```python
from build123d import *

# Parameters (mm, degrees)
F0_W          = 73
F0_H          = 73
F0_W_2        = 56
F0_H_2        = 56
F0_W_3        = 52
F0_H_3        = 52
F1_DEPTH      = 20
F0_W_4        = 76
F0_H_4        = 76
F2_DEPTH      = 3
F3_DEPTH      = 10
F4_W          = 10
F4_H          = 5
F5_DEPTH      = 80
F6_W          = 5
F6_H          = 10
F7_DEPTH      = 80
F8_W          = 8
F8_H          = 5
F9_DEPTH      = 80
F10_W         = 5
F10_H         = 8
F11_DEPTH     = 80
F12_SIZE      = 1
F13_T         = 2.5
F13_T3_DEPTH  = 62
F13_T5_DEPTH  = 62
F13_T7_DEPTH  = 78
F13_T9_DEPTH  = 78
F13_T11_DEPTH = 25


# Not quite as in the source:
# - a shell that OpenCascade refuses in one call is made with other operations: the cavity is built on its own and cut out


with BuildPart() as f1:
    # F0 (on Front) → F1 (new body)
    with BuildSketch(Plane.XZ):
        with Locations((38, 38)):
            Rectangle(F0_W, F0_H)
        with Locations((38, 38)):
            Rectangle(F0_W_2, F0_H_2, mode=Mode.SUBTRACT)
        with Locations((38, 38)):
            Rectangle(F0_W_2, F0_H_2)
        with Locations((38, 38)):
            Rectangle(F0_W_3, F0_H_3, mode=Mode.SUBTRACT)
    extrude(amount=F1_DEPTH)

    # F0 (on Front) → F2 (join)
    with BuildSketch(Plane.XZ):
        with Locations((38, 38)):
            Rectangle(F0_W_4, F0_H_4)
        with Locations((38, 38)):
            Rectangle(F0_W, F0_H, mode=Mode.SUBTRACT)
    extrude(amount=F2_DEPTH)

    # F0 (on Front) → F3 (join)
    with BuildSketch(Plane.XZ):
        with Locations((38, 38)):
            Rectangle(F0_W_4, F0_H_4)
        with Locations((38, 38)):
            Rectangle(F0_W, F0_H, mode=Mode.SUBTRACT)
    extrude(amount=F3_DEPTH)

    # F4 (on Top) → F5 (cut)
    with BuildSketch(Plane.XY):
        with Locations((5, -2.5)):
            Rectangle(F4_W, F4_H)
        with Locations((71, -2.5)):
            Rectangle(F4_W, F4_H)
    extrude(amount=F5_DEPTH, mode=Mode.SUBTRACT)

    # F6 (on Right) → F7 (cut)
    with BuildSketch(Plane.YZ):
        with Locations((-2.5, 5)):
            Rectangle(F6_W, F6_H)
        with Locations((-2.5, 71)):
            Rectangle(F6_W, F6_H)
    extrude(amount=F7_DEPTH, mode=Mode.SUBTRACT)

    # F8 (on Top) → F9 (cut)
    with BuildSketch(Plane.XY):
        with Locations((5.5, -17.5)):
            Rectangle(F8_W, F8_H)
        with Locations((70.5, -17.5)):
            Rectangle(F8_W, F8_H)
    extrude(amount=F9_DEPTH, mode=Mode.SUBTRACT)

    # F10 (on Right) → F11 (cut)
    with BuildSketch(Plane.YZ):
        with Locations((-17.5, 5.5)):
            Rectangle(F10_W, F10_H)
        with Locations((-17.5, 70.5)):
            Rectangle(F10_W, F10_H)
    extrude(amount=F11_DEPTH, mode=Mode.SUBTRACT)

    # F12
    f12_edges = [f1.edges().sort_by_distance(p)[0] for p in [
        (38, -10, 0),
        (0, -10, 38),
        (76, -10, 38),
        (38, -10, 76),
        (66.5, -20, 38),
        (38, -20, 66.5),
        (38, -20, 9.5),
        (9.5, -20, 38),
    ]]
    chamfer(f12_edges, length=F12_SIZE)

    # F13: shell of thickness 2.5, made by hand


with BuildPart() as f13_core1:
    # F13_t2: copy of F1
    add(f1.part)

    # the walls: a layer under each face that stays
    f13_faces = [f13_core1.faces().sort_by_distance(p)[0] for p in [
        (9.5, -17, 38),
        (38, -17, 66.5),
        (10, -19.5, 38),
        (69.2857142857, -15, 69.2857142857),
        (38, -17, 9.5),
        (38, -19.5, 66),
        (66.5, -17, 38),
        (38, -19.5, 10),
        (56.90625, -20, 11.1790123457),
        (1.5, -12.5, 38),
        (38, -12.5, 1.5),
        (74.5, -12.5, 38),
        (38, -12.5, 74.5),
        (66, -19.5, 38),
        (64, -10, 38),
        (38, -10, 64),
        (38, -10, 12),
        (12, -10, 38),
        (40.890625, -10, 1.304526749),
        (11.8666666667, 0, 11.8666666667),
        (38, -9.5, 0.5),
        (0.5, -9.5, 38),
        (75.5, -9.5, 38),
        (38, -9.5, 75.5),
        (66, -2.5, 38),
        (38, -2.5, 10),
        (10, -2.5, 38),
        (38, -2.5, 66),
        (38, -7, 0),
        (0, -7, 38),
        (76, -7, 38),
        (38, -7, 76),
    ]]
    thicken(f13_faces, amount=-F13_T, mode=Mode.SUBTRACT)

    # F13_s4 → F13_t3 (cut)
    with BuildSketch(Plane.XY.offset(7)):
        Polygon((9.475, -15.025), (12, -15), (12, -12.5), (9.5, -12.5), align=None)
        Polygon((66.525, -15.025), (66.5, -12.5), (64, -12.5), (64, -15), align=None)
    extrude(amount=F13_T3_DEPTH, mode=Mode.SUBTRACT)

    # F13_s6 → F13_t5 (cut)
    with BuildSketch(Plane.YZ.offset(7)):
        Polygon((-15.025, 66.525), (-15, 64), (-12.5, 64), (-12.5, 66.5), align=None)
        Polygon((-15.025, 9.475), (-12.5, 9.5), (-12.5, 12), (-15, 12), align=None)
    extrude(amount=F13_T5_DEPTH, mode=Mode.SUBTRACT)

    # F13_s8 → F13_t7 (cut)
    with BuildSketch(Plane.XY.offset(-1)):
        Polygon((1.475, -10.025), (4, -10), (4, -7.5), (1.5, -7.5), align=None)
        Polygon((74.525, -10.025), (72, -10), (72, -7.5), (74.5, -7.5), align=None)
    extrude(amount=F13_T7_DEPTH, mode=Mode.SUBTRACT)

    # F13_s10 → F13_t9 (cut)
    with BuildSketch(Plane.YZ.offset(-1)):
        Polygon((-10.025, 1.475), (-10, 4), (-7.5, 4), (-7.5, 1.5), align=None)
        Polygon((-10.025, 74.525), (-10, 72), (-7.5, 72), (-7.5, 74.5), align=None)
    extrude(amount=F13_T9_DEPTH, mode=Mode.SUBTRACT)

    # F13_s12 → F13_t11 (cut)
    with BuildSketch(Plane.XZ.offset(-2.5)):
        Polygon((63.975, 63.975), (66.5, 64), (66.5, 66.5), (64, 66.5), align=None)
        Polygon((63.975, 12.025), (66.5, 12), (66.5, 9.5), (64, 9.5), align=None)
        Polygon((12.025, 63.975), (12, 66.5), (9.5, 66.5), (9.5, 64), align=None)
        Polygon((12.025, 12.025), (12, 9.5), (9.5, 9.5), (9.5, 12), align=None)
    extrude(amount=F13_T11_DEPTH, mode=Mode.SUBTRACT)


with BuildPart() as f1_1:
    add(f1.part)

    # what is left inside the walls is the cavity
    f13_cavity = [f13_core1.part.solids().sort_by_distance(p)[0] for p in [
        (65.611111, -5.025, 6.9375),
    ]]
    add(f13_cavity, mode=Mode.SUBTRACT)


solid = f1_1.part
```
Can you work these out from the model? Positions are in its coordinate system, mm. A direction names the side the tool comes from. Give positions to 0.01 mm unless a question says otherwise; leave off trailing zeros. Loops run counter-clockwise (first coordinate to the right, second up) from the corner with the lowest first, then second, coordinate; pieces in that order, holes last. Notation, with made-up numbers: M 83.5,23 L 122.5,23 A17 cw 122.5,42 Z; hole C 27,55.25 d7. An arc over 180 degrees is marked long. Use CSV: the item, a comma, the result in double quotes. Start each with the question number.
1. Imagine slicing it at B-B, the plane y = -17. Write out the boundary of the cut face in (x, z).
2. Imagine slicing it at A-A, the plane y = -11.25. Write out the boundary of the cut face in (x, z).
3. If I drill on L1, parallel to Z at x = 60, y = -6; L2, parallel to Z at x = 66, y = -8.5; L3, parallel to X at y = -11.5, z = 18, over which ranges is the centre line in solid material (lowest first)?
4. On a 3-axis mill with a long thin cutter (end or side, diameter ignored), from which of +Z, -Z, +X, -X, +Y, -Y can I reach the whole of each face in a straight line? I mean faces 5 (the face through (12, -10, 38)), 6 (the face through (37, -12, 74.5)), 7 (the face through (9.5, -17, 38)), 8 (the face through (37, -7, 76)), 9 (the face through (38, -9, 9.5)). Say none if no direction works.
5. For P1, Ø4.5, axis at y = -17, z = 30, coming from the -X side; P2, Ø1.5, axis at x = 11, y = -2.5, coming from the +Z side; P3, Ø4, axis at y = -2, z = 12, coming from the -X side, each with a flat end and sliding along its axis, tell me the tip position at first contact or that it passes through.
6. If we mould it in two halves opening along X, with no side actions, what happens to faces 1 (the face through (38, -10, 12)), 2 (the face through (38, -10, 64)), 3 (the face through (38, -3, 10)), 4 (the face through (1.5, -12, 37))? For each: released by +X, released by -X, zero draft, split by the parting line, or undercut.
7. Imagine slicing it at C-C, the plane x = 67.5. Write out the boundary of the cut face in (y, z), plus the area to 4 significant figures.
Response values:
1,outline,"M 9.5,9.5 L 66.5,9.5 L 66.5,66.5 L 9.5,66.5 Z; hole M 12,12 L 64,12 L 64,64 L 12,64 Z"
2,outline,"M 1.5,1.5 L 74.5,1.5 L 74.5,74.5 L 1.5,74.5 Z; M 9.5,9.5 L 66.5,9.5 L 66.5,66.5 L 9.5,66.5 Z; hole M 4,4 L 72,4 L 72,72 L 4,72 Z; hole M 12,12 L 64,12 L 64,64 L 12,64 Z"
3,L1,"0 to 2.5, 9.5 to 12, 64 to 66.5, 73.5 to 76"
3,L2,"0 to 4, 9.5 to 66.5, 72 to 76"
3,L3,"1.5 to 4, 9.5 to 12, 64 to 66.5, 72 to 74.5"
4,face 5,"+Y, -Y"
4,face 6,"+Z, +X, -X, -Y"
4,face 7,"+Z, -Z, -X, -Y"
4,face 8,"+Z, +X, -X, +Y, -Y"
4,face 9,"+Y"
5,P1,"x = 1.5"
5,P2,"z = 66"
5,P3,"x = 10"
6,face 1,"undercut"
6,face 2,"undercut"
6,face 3,"zero draft"
6,face 4,"released by -X"
7,outline,"M -15,1.5 L -10,1.5 L -10,1 L -9,0 L -5,0 L -5,2.5 L -7.5,2.5 L -7.5,4 L -12.5,4 L -12.5,72 L -7.5,72 L -7.5,73.5 L -5,73.5 L -5,76 L -9,76 L -10,75 L -10,74.5 L -15,74.5 Z"
7,area,"226.5 mm^2"
